Part model, mm, in its own coordinate system. A direction names the side the tool comes from. Round coordinates to 2 decimals unless told otherwise and drop trailing zeros. Order: outer loops, then holes, each group sorted by start corner. A loop starts at its lowest first (then second) coordinate and runs counter-clockwise, first axis right, second up. Notation, with made-up numbers: (-40, 82.25) - (-8, 82.25) arc R20 cw to (-8, 101.25) - close; hole circle Ø8 at (86.5, 48.5). An arc over 180 degrees is marked (long way). Return JSON: item names as keys, results as strings. Group by question number.
Item 1: Drop flat-ended pins along their axis: pin 1 (5 mm diameter, centred on y = 3, z = 39, fed in from +X); pin 2 (1 mm diameter, centred on y = 1.5, z = 8.5, fed in from +X); pin 3 (3 mm diameter, centred on x = 6, z = 22.5, fed in from +Y); pin 4 (4.5 mm diameter, centred on y = 0, z = 53.625, fed in from +X). Give the stop position or say it passes through.
Item 2: Probe probe 1 along Z at (x, y) = (-5, 5); probe 2 along Y at (x, z) = (0, 18); probe 3 along Z at (x, y) = (1.25, -1.5) (3 decimals). List the from-to ranges inside material, lowest first.
Item 3: Saw through at C-C on z = 6.5. List the corners of the cut face in (x, y).
Item 4: Two-plate mould, pull along Y, no slides. Class faces 1 (the face through (3, 0, 49)), 2 (the face through (-4.864, 4.461, 20.241)), 3 (the face through (1.5, 0.07, 17.26)): released by +Y, released by -Y, zero draft, split by the parting line, or undercut.
Item 5: Saw through at A-A on y = 0. List the corners of the cut face in (x, z) (3 decimals).
Item 6: Saw through at B-B on x = 0. List the corners of the cut face in (y, z) (3 decimals), and give its area (3 significant figures).
Item 7: Tool access for faces 4 (the face through (-2, -1.9, 51.6)), 5 (the face through (2, -1.9, 51.6)), 6 (the face through (0, -4.375, 51)), 7 (the face through (-3, -6, 47)), 8 (the face through (0, 4.375, 51)): list every direction of +Z, -Z, +X, -X, +Y, -Y with a clear straight run to the whole face (end or side of a thin tool).
```python
from build123d import *

# Parameters (mm, degrees)
SKETCH2_R            = 6.6
EXTERNAL_SHOCK_DEPTH = 39
SHOCK_CHAMFER_SIZE   = 2
SKETCH3_R            = 7.85
CYLINDER_A_DEPTH     = 8
SKETCH4_R            = 6.4
CYLINDER_B_DEPTH     = 2
MOUNTING_BOSS_DEPTH  = 2
SKETCH6_R            = 2.5
MOUNTING_HOLE_DEPTH  = 4
SKETCH7_R            = 1.5
INNER_HOLE_DEPTH     = 35


with BuildPart() as part:
    # Sketch2 → External Shock (new body)
    with BuildSketch(Plane.XY):
        Circle(SKETCH2_R)
    extrude(amount=EXTERNAL_SHOCK_DEPTH)

    # Shock Chamfer
    shock_chamfer_edges = [part.edges().sort_by_distance(p)[0] for p in [
        (-6.6, 0, 0),
    ]]
    chamfer(shock_chamfer_edges, length=SHOCK_CHAMFER_SIZE)

    # Sketch3 → Cylinder A (add)
    with BuildSketch(Plane.XY.offset(39)):
        Circle(SKETCH3_R)
    extrude(amount=CYLINDER_A_DEPTH)

    # Sketch4 → Cylinder B (add)
    with BuildSketch(Plane.XY.offset(47)):
        Circle(SKETCH4_R)
    extrude(amount=CYLINDER_B_DEPTH)

    # Sketch5 → Mounting Boss (add, symmetric)
    with BuildSketch(Plane(origin=(0, 0, 0), x_dir=(0, 0, -1), z_dir=(1, 0, 0))):
        with BuildLine():
            Line((-53.625, -4.375), (-49, -4.375))
            Line((-49, -4.375), (-49, 4.375))
            Line((-49, 4.375), (-53.625, 4.375))
            ThreePointArc((-53.625, 4.375), (-58, 0), (-53.625, -4.375))
        make_face()
    extrude(amount=MOUNTING_BOSS_DEPTH, both=True)

    # Sketch6 → Mounting Hole (cut)
    with BuildSketch(Plane.ZY.offset(2)):
        with Locations((53.625, 0)):
            Circle(SKETCH6_R)
    extrude(amount=-MOUNTING_HOLE_DEPTH, mode=Mode.SUBTRACT)

    # Sketch7 → Inner Hole (cut)
    with BuildSketch(Plane(origin=(0, 0, 0), x_dir=(-1, 0, 0), z_dir=(0, 0, -1))):
        Circle(SKETCH7_R)
    extrude(amount=-INNER_HOLE_DEPTH, mode=Mode.SUBTRACT)


solid = part.part
```
Filled in:
{
 "1": {"pin 1": "stops at x = 7.83", "pin 2": "stops at x = 6.52", "pin 3": "stops at y = 4.83", "pin 4": "passes through"},
 "2": {"probe 1": "z = 39 to 47", "probe 2": "y = -6.6 to -1.5, 1.5 to 6.6", "probe 3": "z = 0 to 51.625, 55.625 to 57.735"},
 "3": {"outline": "circle Ø13.2 at (0, 0); hole circle Ø3 at (0, 0)"},
 "4": {"face 1": "zero draft", "face 2": "split by the parting line", "face 3": "undercut"},
 "5": {"outline": "(-7.85, 39) - (-6.6, 39) - (-6.6, 2) - (-4.6, 0) - (-1.5, 0) - (-1.5, 35) - (1.5, 35) - (1.5, 0) - (4.6, 0) - (6.6, 2) - (6.6, 39) - (7.85, 39) - (7.85, 47) - (6.4, 47) - (6.4, 49) - (2, 49) - (2, 51.125) - (-2, 51.125) - (-2, 49) - (-6.4, 49) - (-6.4, 47) - (-7.85, 47) - close; (-2, 56.125) - (2, 56.125) - (2, 58) - (-2, 58) - close"},
 "6": {"outline": "(-7.85, 39) - (-6.6, 39) - (-6.6, 2) - (-4.6, 0) - (-1.5, 0) - (-1.5, 35) - (1.5, 35) - (1.5, 0) - (4.6, 0) - (6.6, 2) - (6.6, 39) - (7.85, 39) - (7.85, 47) - (6.4, 47) - (6.4, 49) - (4.375, 49) - (4.375, 53.625) arc R4.375 ccw to (-4.375, 53.625) - (-4.375, 49) - (-6.4, 49) - (-6.4, 47) - (-7.85, 47) - close; hole circle Ø5 at (0, 53.625)", "area": "608 mm^2"},
 "7": {"face 4": "+Z, -X, +Y, -Y", "face 5": "+Z, +X, +Y, -Y", "face 6": "+Z, +X, -X, -Y", "face 7": "+Z", "face 8": "+Z, +X, -X, +Y"}
}
